```python
from build123d import *

# Parameters (mm, degrees)
EXTRUDE_1_DEPTH     = 10
SKETCH_2_R          = 20
EXTRUDE_2_DEPTH     = 20
SKETCH_3_R          = 4.5
CUT_EXTRUDE_1_DEPTH = 81
SKETCH_4_R          = 10
CUT_EXTRUDE_2_DEPTH = 65.031242374


with BuildPart() as part:
    # 草图1 → 凸台-拉伸1 (new body)
    with BuildSketch(Plane.XY):
        with BuildLine():
            Line((-30, -40), (30, -40))
            ThreePointArc((30, -40), (37.071067812, -37.071067812), (40, -30))
            Line((40, -30), (40, 30))
            ThreePointArc((40, 30), (37.071067812, 37.071067812), (30, 40))
            Line((30, 40), (-30, 40))
            ThreePointArc((-30, 40), (-37.071067812, 37.071067812), (-40, 30))
            Line((-40, 30), (-40, -30))
            ThreePointArc((-40, -30), (-37.071067812, -37.071067812), (-30, -40))
        make_face()
    extrude(amount=EXTRUDE_1_DEPTH)

    # 草图2 → 凸台-拉伸2 (add)
    with BuildSketch(Plane.XY.offset(10)):
        Circle(SKETCH_2_R)
    extrude(amount=EXTRUDE_2_DEPTH)

    # 草图3 → 切除-拉伸1 (cut, symmetric)
    with BuildSketch(Plane.XY):
        with Locations((30, 30)):
            Circle(SKETCH_3_R)
        with Locations((-30, 30)):
            Circle(SKETCH_3_R)
        with Locations((-30, -30)):
            Circle(SKETCH_3_R)
        with Locations((30, -30)):
            Circle(SKETCH_3_R)
    extrude(amount=CUT_EXTRUDE_1_DEPTH, both=True, mode=Mode.SUBTRACT)

    # 草图4 → 切除-拉伸2 (cut, through all)
    with BuildSketch(Plane.XY.offset(30)):
        Circle(SKETCH_4_R)
    extrude(amount=-CUT_EXTRUDE_2_DEPTH, mode=Mode.SUBTRACT)


solid = part.part
```
Source: CAD feature listing. Evaluate the final solid. Frame: model axes, mm. A direction names the side the tool comes from. Coordinates: 2 decimals unless noted, no trailing zeros. Write each loop counter-clockwise with the first axis right and the second up, starting at its lowest first coordinate (ties: lowest second). Pieces come first, ordered by that corner, then holes. Notation, with made-up numbers: (6, -9) -> (44, -9) arc R21 cw to (44, 21) -> close; hole circle Ø1 at (-23.75, 45). An arc over 180 degrees is marked (long way). Return JSON: item names as keys, results as strings. Group by question number.
1) Contact query for flat-ended pins moving along their axis: P1, Ø8, axis at x = 22, z = 22.5, coming from the -Y side; P2, Ø12, axis at y = 21, z = 20, coming from the +X side; P3, Ø1, axis at x = 7, y = -25.5, coming from the +Z side. Output: stop coordinate, or through.
2) Set-up query: faces 4 (the face through (32.08, -33.99, 5.07)), 5 (the face through (-9.4, 18.3, 10)). Return all of +Z, -Z, +X, -X, +Y, -Y with unobstructed straight access to the full face (end or side cutting, diameter ignored); none if empty.
3) Section query A-A, the plane x = 0. Return loops of the section in (y, z), plus the area to 3 significant figures.
4) Section query D-D, the plane y = 32. Return loops of the section in (x, z), plus the area to 3 significant figures.
5) Ray query, line 1 along Y through (x, z) = (-30, 7.75); line 2 along Y through (x, z) = (0, 15.5). Return the intervals inside material, ascending.
6) Mould query, pull axis Y, two halves, no side actions, for faces 1 (the face through (-37.15, -36.99, 4.93)), 2 (the face through (8, -8, 0)), 3 (the face through (-25.84, -31.72, 4.93)). Classes: +Y half, -Y half, draft (parallel to the pull), parting line (faces both ways), or undercut.
7) Section query C-C, the plane z = 8.75. Return loops of the section in (x, y), plus the area to 3 significant figures.
From the geometry:
{
 "1": {"P1": "y = -8.72", "P2": "x = 13.23", "P3": "z = 10"},
 "2": {"face 4": "+Z, -Z", "face 5": "+Z"},
 "3": {"outline": "(-40, 0) -> (-10, 0) -> (-10, 30) -> (-20, 30) -> (-20, 10) -> (-40, 10) -> close; (10, 0) -> (40, 0) -> (40, 10) -> (20, 10) -> (20, 30) -> (10, 30) -> close", "area": "1,000 mm²"},
 "4": {"outline": "(-39.8, 0) -> (-34.03, 0) -> (-34.03, 10) -> (-39.8, 10) -> close; (-25.97, 0) -> (25.97, 0) -> (25.97, 10) -> (-25.97, 10) -> close; (34.03, 0) -> (39.8, 0) -> (39.8, 10) -> (34.03, 10) -> close", "area": "635 mm²"},
 "5": {"line 1": "-40 to -34.5, -25.5 to 25.5, 34.5 to 40", "line 2": "-20 to -10, 10 to 20"},
 "6": {"face 1": "-Y half", "face 2": "draft", "face 3": "undercut"},
 "7": {"outline": "(-40, -30) arc R10 ccw to (-30, -40) -> (30, -40) arc R10 ccw to (40, -30) -> (40, 30) arc R10 ccw to (30, 40) -> (-30, 40) arc R10 ccw to (-40, 30) -> close; hole circle Ø9 at (-30, -30); hole circle Ø9 at (-30, 30); hole circle Ø20 at (0, 0); hole circle Ø9 at (30, -30); hole circle Ø9 at (30, 30)", "area": "5,750 mm²"}
}
